Autodesk Inventor part; units mm, degrees
ref_plane "YZ Plane" through (0, 0, 0) normal (1, 0, 0) x (0, 1, 0)
ref_plane "XZ Plane" through (0, 0, 0) normal (0, 1, 0) x (-1, 0, 0)
ref_plane "XY Plane" through (0, 0, 0) normal (0, 0, 1) x (1, 0, 0)
sketch "スケッチ1" plane through (0, 0, 0) normal (0, 0, 1) x (1, 0, 0)
  circle A0 centre (0, 0) radius 2.5
  dimension "d0" = 5
extrude "押し出し1" add sketch "スケッチ1" along normal blind 6
sketch "スケッチ2" plane through (0, 0, 6) normal (0, 0, 1) x (1, 0, 0)
  circle A0 centre (0, 0) radius 2.5
  circle A1 centre (0, 0) radius 5
  dimension "d3" = 10
extrude "押し出し2" add sketch "スケッチ2" along normal blind 2.8 contours A0 | A1
thread "ねじ1"
chamfer "面取り1" distance 2.5 angle 45 1 edges at (-5, 0, 6)
sketch "スケッチ4" plane through (0, 0, 0) normal (0, 0, -1) x (-1, 0, 0)
  circle A0 centre (0, 0) radius 2.5
  dimension "d16" = 5
extrude "押し出し4" add sketch "スケッチ4" along normal blind 9.7
properties part number "SB　M5 18mm 皿ネジ" material "Stainless Steel, 440C"
Work out the finished part from the listing and answer in its coordinate system (mm). Coordinates: 2 decimals unless noted, no trailing zeros. Order: outer loops, then holes, each group sorted by start corner. A loop starts at its lowest first (then second) coordinate and runs counter-clockwise, first axis right, second up. Notation, with made-up numbers: (-26, 56) - (8, 56) arc R18 ccw to (8, 71) - close; hole circle Ø8 at (-32, -12.5). An arc over 180 degrees is marked (long way). Put each result on its own line as item: value. Start each with the question number.
1) Find the intervals of material crossed by line 1 (Z direction, x = -2, y = 2.25); line 2 (Y direction, x = 2.5, z = 6.75); line 3 (Z direction, x = -3.5, y = 2), in increasing order. Write a range as from..to.
2) Find section D-D (z = 6.75). Give the vertices of the cut face in (x, y), plus the area to 3 significant figures.
3) Find section C-C (z = -6.5). Give the vertices of the cut face in (x, y).
4) Flat-ended cylindrical pins translate along their axes: pin 1 (3 mm diameter, centred on x = -0.5, z = -6, fed in from +Y); pin 2 (1.5 mm diameter, centred on x = -4, z = -2, fed in from -Y); pin 3 (3 mm diameter, centred on x = -2.5, z = 4.5, fed in from +Y). Find the tip coordinate at first contact, or state that the pin passes through.
Results list:
1. line 1: z = 6.51..8.8
1. line 2: y = -2.08..2.08
1. line 3: z = 7.53..8.8
2. outline: circle Ø6.5 at (0, 0)
2. area: 33.2 mm^2
3. outline: circle Ø5 at (0, 0)
4. pin 1: stops at y = 2.5
4. pin 2: passes through
4. pin 3: stops at y = 2.29
